The listing builds one solid part. Answer for the finished solid, in the listing's coordinates (mm). Face numbers are marked on the shaded views. Round coordinates to 2 decimals unless told otherwise and drop trailing zeros. Loops run counter-clockwise (first coordinate to the right, second up) from the corner with the lowest first, then second, coordinate; pieces in that order, holes last. Notation, with made-up numbers: (29.5, -9.75) -> (52.5, -9.75) arc R29 cw to (52.5, 28.25) -> close; hole circle Ø8 at (7, 49). An arc over 180 degrees is marked (long way). Use a Markdown table: item, result. Add a question column.
Q1. Given pin 1 Ø3 at (x, y) = (-1.5, 68) entering from +Z; pin 2 Ø8 at (x, y) = (2.5, -71) entering from -Z; pin 3 Ø10 at (x, z) = (61, 28) entering from +Y; pin 4 Ø1.5 at (x, z) = (59.5, 20.5) entering from +Y, each flat-ended and moving along its own axis, determine where each tip first touches the part or whether it passes through.
Q2. Section A-A on y = -82.5 is taken. Give the vertices of the cut face in (x, z), then the cut area to 3 significant figures.
Q3. For a pull along Z with two mould halves and no side action, classify the marked faces 1, 2 and 3 as released by +Z, released by -Z, zero draft, split by the parting line, or undercut.
Q4. Section C-C on y = 0 is taken. Give the vertices of the cut face in (x, z).
Q5. Consider line 1 (Z direction, x = -2.5, y = 38.5); line 2 (X direction, y = -72, z = 111); line 3 (Y direction, x = -73, z = 25). Determine where each line is inside the solid, lowest interval first.
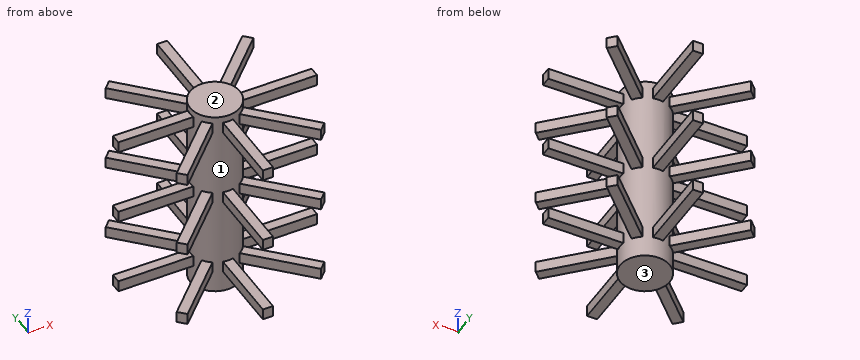
from build123d import *

# Parameters (mm, degrees)
SKETCH1_R                  = 25.4
BOSS_EXTRUDE1_DEPTH        = 203.31507114
SKETCH3_W                  = 11.610363297
SKETCH3_H                  = 10.2808948
BOSS_EXTRUDE3_DEPTH        = 101.6
CIRPATTERN4_COUNT          = 8
LPATTERN1_COUNT            = 3
LPATTERN1_PITCH            = 81.28
LPATTERN1_COPY_1_SKETCH_W  = 11.610363297
LPATTERN1_COPY_1_SKETCH_H  = 10.2808948
LPATTERN1_COPY_1_DEPTH     = 101.6
LPATTERN1_COPY_2_SKETCH_W  = 11.610363297
LPATTERN1_COPY_2_SKETCH_H  = 10.2808948
LPATTERN1_COPY_2_DEPTH     = 101.6
LPATTERN1_COPY_3_SKETCH_W  = 11.610363297
LPATTERN1_COPY_3_SKETCH_H  = 10.2808948
LPATTERN1_COPY_3_DEPTH     = 101.6
LPATTERN1_COPY_4_SKETCH_W  = 11.610363297
LPATTERN1_COPY_4_SKETCH_H  = 10.2808948
LPATTERN1_COPY_4_DEPTH     = 101.6
LPATTERN1_COPY_5_SKETCH_W  = 11.610363297
LPATTERN1_COPY_5_SKETCH_H  = 10.2808948
LPATTERN1_COPY_5_DEPTH     = 101.6
LPATTERN1_COPY_6_SKETCH_W  = 11.610363297
LPATTERN1_COPY_6_SKETCH_H  = 10.2808948
LPATTERN1_COPY_6_DEPTH     = 101.6
LPATTERN1_COPY_7_SKETCH_W  = 11.610363297
LPATTERN1_COPY_7_SKETCH_H  = 10.2808948
LPATTERN1_COPY_7_DEPTH     = 101.6
LPATTERN1_COPY_8_SKETCH_W  = 11.610363297
LPATTERN1_COPY_8_SKETCH_H  = 10.2808948
LPATTERN1_COPY_8_DEPTH     = 101.6
LPATTERN1_COPY_9_SKETCH_W  = 11.610363297
LPATTERN1_COPY_9_SKETCH_H  = 10.2808948
LPATTERN1_COPY_9_DEPTH     = 101.6
LPATTERN1_COPY_10_SKETCH_W = 11.610363297
LPATTERN1_COPY_10_SKETCH_H = 10.2808948
LPATTERN1_COPY_10_DEPTH    = 101.6
LPATTERN1_COPY_11_SKETCH_W = 11.610363297
LPATTERN1_COPY_11_SKETCH_H = 10.2808948
LPATTERN1_COPY_11_DEPTH    = 101.6
LPATTERN1_COPY_12_SKETCH_W = 11.610363297
LPATTERN1_COPY_12_SKETCH_H = 10.2808948
LPATTERN1_COPY_12_DEPTH    = 101.6
LPATTERN1_COPY_13_SKETCH_W = 11.610363297
LPATTERN1_COPY_13_SKETCH_H = 10.2808948
LPATTERN1_COPY_13_DEPTH    = 101.6
LPATTERN1_COPY_14_SKETCH_W = 11.610363297
LPATTERN1_COPY_14_SKETCH_H = 10.2808948
LPATTERN1_COPY_14_DEPTH    = 101.6


with BuildPart() as part:
    # Sketch1 → Boss-Extrude1 (new body)
    with BuildSketch(Plane.XY):
        with Locations(Location((0, 0, 0), (0, 0, 180))):
            Circle(SKETCH1_R)
    extrude(amount=BOSS_EXTRUDE1_DEPTH)

    # Sketch3 → Boss-Extrude3 (add)
    with BuildSketch(Plane(origin=(0, 0, 0), x_dir=(0, 0, -1), z_dir=(1, 0, 0))):
        with Locations((-190.503475636, 0)):
            Rectangle(SKETCH3_W, SKETCH3_H)
    boss_extrude3 = extrude(amount=BOSS_EXTRUDE3_DEPTH)

    # CirPattern4: Boss-Extrude3 ×8 about axis
    cirpattern4_axis = Axis((0, 0, 0), (0, 0, 1))
    for i in range(1, CIRPATTERN4_COUNT):
        add(boss_extrude3.rotate(cirpattern4_axis, i * 360 / CIRPATTERN4_COUNT))

    # LPattern1: Boss-Extrude3 ×3
    with Locations(*[(0, 0, -i * LPATTERN1_PITCH) for i in range(1, LPATTERN1_COUNT)]):
        add(boss_extrude3)

    # LPattern1 copy 1 sketch → LPattern1 copy 1 (add)
    with BuildSketch(Plane(origin=(0, 0, -81.28), x_dir=(0, 0, -1), z_dir=(0.7071067811865476, 0.7071067811865475, 0))):
        with Locations((-190.503475636, 0)):
            Rectangle(LPATTERN1_COPY_1_SKETCH_W, LPATTERN1_COPY_1_SKETCH_H)
    extrude(amount=LPATTERN1_COPY_1_DEPTH)

    # LPattern1 copy 2 sketch → LPattern1 copy 2 (add)
    with BuildSketch(Plane(origin=(0, 0, -162.56), x_dir=(0, 0, -1), z_dir=(0.7071067811865476, 0.7071067811865475, 0))):
        with Locations((-190.503475636, 0)):
            Rectangle(LPATTERN1_COPY_2_SKETCH_W, LPATTERN1_COPY_2_SKETCH_H)
    extrude(amount=LPATTERN1_COPY_2_DEPTH)

    # LPattern1 copy 3 sketch → LPattern1 copy 3 (add)
    with BuildSketch(Plane(origin=(0, 0, -81.28), x_dir=(0, 0, -1), z_dir=(0, 1, 0))):
        with Locations((-190.503475636, 0)):
            Rectangle(LPATTERN1_COPY_3_SKETCH_W, LPATTERN1_COPY_3_SKETCH_H)
    extrude(amount=LPATTERN1_COPY_3_DEPTH)

    # LPattern1 copy 4 sketch → LPattern1 copy 4 (add)
    with BuildSketch(Plane(origin=(0, 0, -162.56), x_dir=(0, 0, -1), z_dir=(0, 1, 0))):
        with Locations((-190.503475636, 0)):
            Rectangle(LPATTERN1_COPY_4_SKETCH_W, LPATTERN1_COPY_4_SKETCH_H)
    extrude(amount=LPATTERN1_COPY_4_DEPTH)

    # LPattern1 copy 5 sketch → LPattern1 copy 5 (add)
    with BuildSketch(Plane(origin=(0, 0, -81.28), x_dir=(0, 0, -1), z_dir=(-0.7071067811865475, 0.7071067811865476, 0))):
        with Locations((-190.503475636, 0)):
            Rectangle(LPATTERN1_COPY_5_SKETCH_W, LPATTERN1_COPY_5_SKETCH_H)
    extrude(amount=LPATTERN1_COPY_5_DEPTH)

    # LPattern1 copy 6 sketch → LPattern1 copy 6 (add)
    with BuildSketch(Plane(origin=(0, 0, -162.56), x_dir=(0, 0, -1), z_dir=(-0.7071067811865475, 0.7071067811865476, 0))):
        with Locations((-190.503475636, 0)):
            Rectangle(LPATTERN1_COPY_6_SKETCH_W, LPATTERN1_COPY_6_SKETCH_H)
    extrude(amount=LPATTERN1_COPY_6_DEPTH)

    # LPattern1 copy 7 sketch → LPattern1 copy 7 (add)
    with BuildSketch(Plane(origin=(0, 0, -81.28), x_dir=(0, 0, -1), z_dir=(-1, 0, 0))):
        with Locations((-190.503475636, 0)):
            Rectangle(LPATTERN1_COPY_7_SKETCH_W, LPATTERN1_COPY_7_SKETCH_H)
    extrude(amount=LPATTERN1_COPY_7_DEPTH)

    # LPattern1 copy 8 sketch → LPattern1 copy 8 (add)
    with BuildSketch(Plane(origin=(0, 0, -162.56), x_dir=(0, 0, -1), z_dir=(-1, 0, 0))):
        with Locations((-190.503475636, 0)):
            Rectangle(LPATTERN1_COPY_8_SKETCH_W, LPATTERN1_COPY_8_SKETCH_H)
    extrude(amount=LPATTERN1_COPY_8_DEPTH)

    # LPattern1 copy 9 sketch → LPattern1 copy 9 (add)
    with BuildSketch(Plane(origin=(0, 0, -81.28), x_dir=(0, 0, -1), z_dir=(-0.7071067811865477, -0.7071067811865475, 0))):
        with Locations((-190.503475636, 0)):
            Rectangle(LPATTERN1_COPY_9_SKETCH_W, LPATTERN1_COPY_9_SKETCH_H)
    extrude(amount=LPATTERN1_COPY_9_DEPTH)

    # LPattern1 copy 10 sketch → LPattern1 copy 10 (add)
    with BuildSketch(Plane(origin=(0, 0, -162.56), x_dir=(0, 0, -1), z_dir=(-0.7071067811865477, -0.7071067811865475, 0))):
        with Locations((-190.503475636, 0)):
            Rectangle(LPATTERN1_COPY_10_SKETCH_W, LPATTERN1_COPY_10_SKETCH_H)
    extrude(amount=LPATTERN1_COPY_10_DEPTH)

    # LPattern1 copy 11 sketch → LPattern1 copy 11 (add)
    with BuildSketch(Plane(origin=(0, 0, -81.28), x_dir=(0, 0, -1), z_dir=(0, -1, 0))):
        with Locations((-190.503475636, 0)):
            Rectangle(LPATTERN1_COPY_11_SKETCH_W, LPATTERN1_COPY_11_SKETCH_H)
    extrude(amount=LPATTERN1_COPY_11_DEPTH)

    # LPattern1 copy 12 sketch → LPattern1 copy 12 (add)
    with BuildSketch(Plane(origin=(0, 0, -162.56), x_dir=(0, 0, -1), z_dir=(0, -1, 0))):
        with Locations((-190.503475636, 0)):
            Rectangle(LPATTERN1_COPY_12_SKETCH_W, LPATTERN1_COPY_12_SKETCH_H)
    extrude(amount=LPATTERN1_COPY_12_DEPTH)

    # LPattern1 copy 13 sketch → LPattern1 copy 13 (add)
    with BuildSketch(Plane(origin=(0, 0, -81.28), x_dir=(0, 0, -1), z_dir=(0.7071067811865474, -0.7071067811865477, 0))):
        with Locations((-190.503475636, 0)):
            Rectangle(LPATTERN1_COPY_13_SKETCH_W, LPATTERN1_COPY_13_SKETCH_H)
    extrude(amount=LPATTERN1_COPY_13_DEPTH)

    # LPattern1 copy 14 sketch → LPattern1 copy 14 (add)
    with BuildSketch(Plane(origin=(0, 0, -162.56), x_dir=(0, 0, -1), z_dir=(0.7071067811865474, -0.7071067811865477, 0))):
        with Locations((-190.503475636, 0)):
            Rectangle(LPATTERN1_COPY_14_SKETCH_W, LPATTERN1_COPY_14_SKETCH_H)
    extrude(amount=LPATTERN1_COPY_14_DEPTH)


solid = part.part
Checked values:
| question | item | result |
|---|---|---|
| 1 | pin 1 | stops at z = 196.31 |
| 1 | pin 2 | stops at z = 22.14 |
| 1 | pin 3 | stops at y = 73.27 |
| 1 | pin 4 | passes through |
| 2 | outline | (-5.14, 22.14) -> (5.14, 22.14) -> (5.14, 33.75) -> (-5.14, 33.75) -> close; (-5.14, 103.42) -> (5.14, 103.42) -> (5.14, 115.03) -> (-5.14, 115.03) -> close; (-5.14, 184.7) -> (5.14, 184.7) -> (5.14, 196.31) -> (-5.14, 196.31) -> close |
| 2 | area | 358 mm2 |
| 3 | face 1 | undercut |
| 3 | face 2 | released by +Z |
| 3 | face 3 | released by -Z |
| 4 | outline | (-101.6, 22.14) -> (-25.4, 22.14) -> (-25.4, 0) -> (25.4, 0) -> (25.4, 22.14) -> (101.6, 22.14) -> (101.6, 33.75) -> (25.4, 33.75) -> (25.4, 103.42) -> (101.6, 103.42) -> (101.6, 115.03) -> (25.4, 115.03) -> (25.4, 184.7) -> (101.6, 184.7) -> (101.6, 196.31) -> (25.4, 196.31) -> (25.4, 203.32) -> (-25.4, 203.32) -> (-25.4, 196.31) -> (-101.6, 196.31) -> (-101.6, 184.7) -> (-25.4, 184.7) -> (-25.4, 115.03) -> (-101.6, 115.03) -> (-101.6, 103.42) -> (-25.4, 103.42) -> (-25.4, 33.75) -> (-101.6, 33.75) -> close |
| 5 | line 1 | z = 22.14 to 33.75, 103.42 to 115.03, 184.7 to 196.31 |
| 5 | line 2 | x = -71.68 to -64.73, -5.14 to 5.14, 64.73 to 71.68 |
| 5 | line 3 | y = -70.68 to -65.73, -5.14 to 5.14, 65.73 to 70.68 |
